The model under review builds one solid part; all positions refer to its coordinate system, in mm. A direction names the side the tool comes from. Coordinates: 2 decimals unless noted, no trailing zeros. Loops run counter-clockwise (first coordinate to the right, second up) from the corner with the lowest first, then second, coordinate; pieces in that order, holes last. Notation, with made-up numbers: (-2, -39.75) - (48, -39.75) arc R19 cw to (48, -28.75) - close; hole circle Ø2 at (40, 13). An arc over 180 degrees is marked (long way). Answer in a Markdown table with one row per item. Add a question column.
(1) Mouldability with a two-part tool opening along X and no side actions: class faces 3 (the cylindrical face through (122.163, 26.783, 71.869)), 4 (the flat face through (124.6, -16.1, 69.5)) as +X half, -X half, draft (parallel to the pull), parting line (faces both ways), or undercut.
(2) For P1, Ø5, axis at x = 124.5, z = 66.5, coming from the +Y side; P2, Ø1.5, axis at y = 28.5, z = 68.5, coming from the +X side; P3, Ø3, axis at x = 123.75, y = 28, coming from the +Z side; P4, Ø1, axis at x = 166, z = 71, coming from the +Y side, all flat-tipped, find the tip position at first contact; note any pin that passes through.
(3) We need section B-B on y = -18.5. Write out the cut boundary in (x, z), plus the area to 3 significant figures.
(4) Machinability: for faces 1 (the flat face through (123.7, -10.2, 74.82)), 2 (the flat face through (144, -8, 69)), which of the approach directions +Z, -Z, +X, -X, +Y, -Y give a long, thin tool a straight path to every point of the face, cutting with its end or side? Answer none if there is none.
(5) We need section A-A on z = 71.5. Give the number of separate pieces and of enclosed holes in the cut face, plus the area to 3 significant figures.
(6) For line 1 along X through (y, z) = (28, 72.5); line 2 along X through (y, z) = (28, 71.7); line 3 along Y through (x, z) = (123.75, 72.4), list the stretches that pass through material, from the lowest coordinate up.
from build123d import *

# Parameters (mm, degrees)
CYLINDER180_R             = 2
CYLINDER180_DEPTH         = 10
CYLINDER181_R             = 2
CYLINDER181_DEPTH         = 10
CYLINDER182_R             = 2
CYLINDER182_DEPTH         = 10
CYLINDER183_R             = 2
CYLINDER183_DEPTH         = 10
CYLINDER170_R             = 2
CYLINDER170_DEPTH         = 10
CYLINDER171_R             = 2
CYLINDER171_DEPTH         = 10
CYLINDER172_R             = 2
CYLINDER172_DEPTH         = 10
CYLINDER169_R             = 2
CYLINDER169_DEPTH         = 10
FUSION111_PLACEMENT_ANGLE = 45
CYLINDER175_R             = 5.5
CYLINDER175_DEPTH         = 1
CYLINDER176_R             = 5
CYLINDER176_DEPTH         = 5.82
CYLINDER177_R             = 5
CYLINDER177_DEPTH         = 5.82
CYLINDER178_R             = 5
CYLINDER178_DEPTH         = 5.82
CYLINDER179_R             = 5
CYLINDER179_DEPTH         = 5.82
CYLINDER173_R             = 40
CYLINDER173_DEPTH         = 4.5
CYLINDER174_R             = 24
CYLINDER174_DEPTH         = 7


with BuildPart() as cylinder180:
    # Cylinder180 → Cylinder180 (new body)
    with BuildSketch(Plane(origin=(0, -21, 0), x_dir=(1, 0, 0), z_dir=(0, 0, 1))):
        Circle(CYLINDER180_R)
    extrude(amount=CYLINDER180_DEPTH)


with BuildPart() as m3heatsetcuts031:
    # Cylinder181 → Cylinder181 (new body)
    with BuildSketch(Plane(origin=(20.5, -21, 0), x_dir=(1, 0, 0), z_dir=(0, 0, 1))):
        Circle(CYLINDER181_R)
    extrude(amount=CYLINDER181_DEPTH)

    # Fusion118: union Cylinder180
    add(cylinder180.part)


with BuildPart() as m3heatsetcuts031_1:
    # Fusion118 placement: moved
    add(m3heatsetcuts031.part.moved(Location((-5, 39, 70))))


with BuildPart() as cylinder182:
    # Cylinder182 → Cylinder182 (new body)
    with BuildSketch(Plane(origin=(0, -21, 0), x_dir=(1, 0, 0), z_dir=(0, 0, 1))):
        Circle(CYLINDER182_R)
    extrude(amount=CYLINDER182_DEPTH)


with BuildPart() as m3heatsetcuts030:
    # Cylinder183 → Cylinder183 (new body)
    with BuildSketch(Plane(origin=(20.5, -21, 0), x_dir=(1, 0, 0), z_dir=(0, 0, 1))):
        Circle(CYLINDER183_R)
    extrude(amount=CYLINDER183_DEPTH)

    # Fusion119: union Cylinder182
    add(cylinder182.part)


with BuildPart() as m3heatsetcuts030_1:
    # Fusion119 placement: moved
    add(m3heatsetcuts030.part.moved(Location((-5, 3, 70))))

    # Fusion117: union m3HeatSetCuts031
    add(m3heatsetcuts031_1.part)


with BuildPart() as m3heatsetcuts030_2:
    # Fusion117 placement: moved
    add(m3heatsetcuts030_1.part.moved(Location((128.75, 10, -1))))


with BuildPart() as obj1:
    # Cylinder170 → Cylinder170 (new body)
    with BuildSketch(Plane(origin=(35, 0, 65), x_dir=(1, 0, 0), z_dir=(0, 0, 1))):
        Circle(CYLINDER170_R)
    extrude(amount=CYLINDER170_DEPTH)


with BuildPart() as obj2:
    # Cylinder171 → Cylinder171 (new body)
    with BuildSketch(Plane(origin=(0, 35, 65), x_dir=(1, 0, 0), z_dir=(0, 0, 1))):
        Circle(CYLINDER171_R)
    extrude(amount=CYLINDER171_DEPTH)


with BuildPart() as obj3:
    # Cylinder172 → Cylinder172 (new body)
    with BuildSketch(Plane(origin=(0, -35, 65), x_dir=(1, 0, 0), z_dir=(0, 0, 1))):
        Circle(CYLINDER172_R)
    extrude(amount=CYLINDER172_DEPTH)


with BuildPart() as fusion120:
    # Cylinder169 → Cylinder169 (new body)
    with BuildSketch(Plane(origin=(-35, 0, 65), x_dir=(1, 0, 0), z_dir=(0, 0, 1))):
        Circle(CYLINDER169_R)
    extrude(amount=CYLINDER169_DEPTH)

    # Fusion111: union obj1, obj2, obj3
    add(obj1.part)
    add(obj2.part)
    add(obj3.part)


with BuildPart() as fusion120_1:
    # Fusion111 placement: moved
    add(fusion120.part.moved(Location((0, -374, -75))).rotate(Axis((0, -374, -75), (0, 0, -1)), FUSION111_PLACEMENT_ANGLE))

    # Fusion120: union m3HeatSetCuts030
    add(m3heatsetcuts030_2.part)


with BuildPart() as cylinder175:
    # Cylinder175 → Cylinder175 (new body)
    with BuildSketch(Plane(origin=(134, 32.6, 65), x_dir=(1, 0, 0), z_dir=(0, 0, 1))):
        Circle(CYLINDER175_R)
    extrude(amount=CYLINDER175_DEPTH)


with BuildPart() as cylinder176:
    # Cylinder176 → Cylinder176 (new body)
    with BuildSketch(Plane(origin=(0, -21, 0), x_dir=(1, 0, 0), z_dir=(0, 0, 1))):
        Circle(CYLINDER176_R)
    extrude(amount=CYLINDER176_DEPTH)


with BuildPart() as m3heatsetcuts027:
    # Cylinder177 → Cylinder177 (new body)
    with BuildSketch(Plane(origin=(20.5, -21, 0), x_dir=(1, 0, 0), z_dir=(0, 0, 1))):
        Circle(CYLINDER177_R)
    extrude(amount=CYLINDER177_DEPTH)

    # Fusion112: union Cylinder176
    add(cylinder176.part)


with BuildPart() as m3heatsetcuts027_1:
    # Fusion112 placement: moved
    add(m3heatsetcuts027.part.moved(Location((-5, 39, 70))))


with BuildPart() as cylinder178:
    # Cylinder178 → Cylinder178 (new body)
    with BuildSketch(Plane(origin=(0, -21, 0), x_dir=(1, 0, 0), z_dir=(0, 0, 1))):
        Circle(CYLINDER178_R)
    extrude(amount=CYLINDER178_DEPTH)


with BuildPart() as m3heatsetcuts029:
    # Cylinder179 → Cylinder179 (new body)
    with BuildSketch(Plane(origin=(20.5, -21, 0), x_dir=(1, 0, 0), z_dir=(0, 0, 1))):
        Circle(CYLINDER179_R)
    extrude(amount=CYLINDER179_DEPTH)

    # Fusion113: union Cylinder178
    add(cylinder178.part)


with BuildPart() as m3heatsetcuts029_1:
    # Fusion113 placement: moved
    add(m3heatsetcuts029.part.moved(Location((-5, 3, 70))))

    # Fusion114: union m3HeatSetCuts027
    add(m3heatsetcuts027_1.part)


with BuildPart() as m3heatsetcuts029_2:
    # Fusion114 placement: moved
    add(m3heatsetcuts029_1.part.moved(Location((128.75, 10, -1))))


with BuildPart() as base015:
    # Cylinder173 → Cylinder173 (new body)
    with BuildSketch(Plane(origin=(136, 0, 65), x_dir=(1, 0, 0), z_dir=(0, 0, 1))):
        Circle(CYLINDER173_R)
    extrude(amount=CYLINDER173_DEPTH)


with BuildPart() as basecut004:
    # Cylinder174 → Cylinder174 (new body)
    with BuildSketch(Plane(origin=(5, 0, 74), x_dir=(1, 0, 0), z_dir=(0, 0, 1))):
        Circle(CYLINDER174_R)
    extrude(amount=CYLINDER174_DEPTH)


with BuildPart() as cut059:
    # Sphere006 → Sphere006 (revolve)
    with BuildSketch(Plane(origin=(5, 0, 74), x_dir=(1, 0, 0), z_dir=(0, -1, 0))):
        with BuildLine():
            ThreePointArc((27.5, 0), (27.349352, 2.874533), (26.899059, 5.717571))
            Line((26.899059, 5.717571), (0, 5.717571))
            Line((0, 5.717571), (0, 0))
            Line((0, 0), (27.5, 0))
        make_face()
    revolve(axis=Axis((5, 0, 74), (0, 0, 1)))

    # Cut058: cut baseCut004
    add(basecut004.part, mode=Mode.SUBTRACT)


with BuildPart() as cut059_1:
    # Cut058 placement: moved
    add(cut059.part.moved(Location((131, 0, -5))))

    # Fusion115: union base015
    add(base015.part)


with BuildPart() as cut059_2:
    # Fusion115 placement: moved
    add(cut059_1.part.moved(Location((-2, 10, 0))))

    # Fusion116: union Cylinder175, m3HeatSetCuts029
    add(cylinder175.part)
    add(m3heatsetcuts029_2.part)

    # Cut059: cut Fusion120
    add(fusion120_1.part, mode=Mode.SUBTRACT)


solid = cut059_2.part
Outcome:
| question | item | result |
|---|---|---|
| 1 | face 3 | undercut |
| 1 | face 4 | draft |
| 2 | P1 | y = 49.38 |
| 2 | P2 | x = 169.85 |
| 2 | P3 | z = 69 |
| 2 | P4 | through |
| 3 | outline | (105.93, 65) - (162.07, 65) - (162.07, 69.5) - (105.93, 69.5) - close |
| 3 | area | 253 mm² |
| 4 | face 1 | +Z, +X, -X, +Y, -Y |
| 4 | face 2 | +Z |
| 5 | separate pieces | 1 |
| 5 | enclosed holes | 5 |
| 5 | area | 771 mm² |
| 6 | line 1 | 113.51 to 118.13, 118.75 to 121.75, 125.75 to 128.75, 139.25 to 142.25, 146.25 to 149.25, 149.87 to 154.49 |
| 6 | line 2 | 113.39 to 118.13, 118.75 to 121.75, 125.75 to 128.75, 139.25 to 142.25, 146.25 to 149.25, 149.87 to 154.61 |
| 6 | line 3 | -15.29 to -10, -6 to -3, 23 to 26, 30 to 35.29 |
